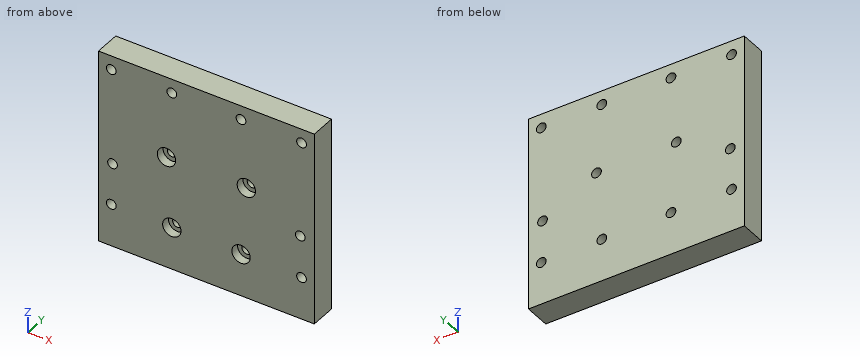
from build123d import *

# Parameters (mm, degrees)
SKETCH_W        = 100
SKETCH_H        = 90
PAD_DEPTH       = 12
SKETCH001_R     = 2.25
POCKET_DEPTH    = 12.001
SKETCH002_R     = 4.25
POCKET001_DEPTH = 4


with BuildPart() as part:
    # Sketch → Pad (new body)
    with BuildSketch(Plane.XZ):
        Rectangle(SKETCH_W, SKETCH_H)
    extrude(amount=PAD_DEPTH)

    # Sketch001 → Pocket (cut, through all)
    with BuildSketch(Plane.XZ.offset(12)):
        with Locations((-44.075, -25.33)):
            Circle(SKETCH001_R)
        with Locations((-43.5, -5.85)):
            Circle(SKETCH001_R)
        with Locations((-16.025, -25.33)):
            Circle(SKETCH001_R)
        with Locations((16.025, -25.33)):
            Circle(SKETCH001_R)
        with Locations((44.075, -25.33)):
            Circle(SKETCH001_R)
        with Locations((43.5, -5.85)):
            Circle(SKETCH001_R)
        with Locations((-44.075, 38.53)):
            Circle(SKETCH001_R)
        with Locations((-16.025, 38.53)):
            Circle(SKETCH001_R)
        with Locations((16.025, 38.53)):
            Circle(SKETCH001_R)
        with Locations((44.075, 38.53)):
            Circle(SKETCH001_R)
        with Locations((-18.5, 7.1)):
            Circle(SKETCH001_R)
        with Locations((18.5, 7.1)):
            Circle(SKETCH001_R)
    extrude(amount=-POCKET_DEPTH, mode=Mode.SUBTRACT)

    # Sketch002 → Pocket001 (cut)
    with BuildSketch(Plane.XZ.offset(12)):
        with Locations((-16.025, -25.33)):
            Circle(SKETCH002_R)
        with Locations((16.025, -25.33)):
            Circle(SKETCH002_R)
        with Locations((-18.5, 7.1)):
            Circle(SKETCH002_R)
        with Locations((18.5, 7.1)):
            Circle(SKETCH002_R)
    extrude(amount=-POCKET001_DEPTH, mode=Mode.SUBTRACT)


solid = part.part
For this review, take the finished solid that the model builds, in its own axes (mm). Round coordinates to 2 decimals unless told otherwise and drop trailing zeros. Loops run counter-clockwise (first coordinate to the right, second up) from the corner with the lowest first, then second, coordinate; pieces in that order, holes last. Notation, with made-up numbers: (50.25, 14) - (72.25, 14) arc R16 ccw to (72.25, 40) - close; hole circle Ø2 at (-15.5, -15.75). An arc over 180 degrees is marked (long way). Answer as CSV lines item,"result".
(1) Consider section B-B on y = -10.75. Give the number of separate pieces and of enclosed holes in the cut face, then the cut area to 3 significant figures.
Checked values:
separate pieces,"1"
enclosed holes,"12"
area,"8,650 mm2"
(2) Insertion check: P1, Ø3.5, axis at x = 44.075, z = 38.53, coming from the -Y side; P2, Ø2.5, axis at x = -20.5, z = 9, coming from the -Y side. Each pin has a flat end and moves straight along its axis. Give the tip position at first contact, or say it passes through.
Checked values:
P1,"passes through"
P2,"stops at y = -8"
(3) Wall thickness on line 1 (X direction, y = -9.25, z = -27); line 2 (Z direction, x = 18.5, y = -3.75); line 3 (Z direction, x = 18, y = -1.25): over which ranges is each line inside the solid? List them lowest first.
Checked values:
line 1,"x = -50 to -45.58, -42.57 to -19.93, -12.12 to 12.12, 19.93 to 42.57, 45.58 to 50"
line 2,"z = -45 to 4.85, 9.35 to 45"
line 3,"z = -45 to -26.41, -24.25 to 4.91, 9.29 to 37.45, 39.61 to 45"
(4) Consider section C-C on z = -5.85. Give the boundary of the cut face in (x, y).
Checked values:
outline,"(-50, -12) - (-45.75, -12) - (-45.75, 0) - (-50, 0) - close; (-41.25, -12) - (41.25, -12) - (41.25, 0) - (-41.25, 0) - close; (45.75, -12) - (50, -12) - (50, 0) - (45.75, 0) - close"
(5) Consider section A-A on z = -25.33. Give the boundary of the cut face in (x, y) (3 decimals).
Checked values:
outline,"(-50, -12) - (-46.325, -12) - (-46.325, 0) - (-50, 0) - close; (-41.825, -12) - (-20.275, -12) - (-20.275, -8) - (-18.275, -8) - (-18.275, 0) - (-41.825, 0) - close; (-13.775, -8) - (-11.775, -8) - (-11.775, -12) - (11.775, -12) - (11.775, -8) - (13.775, -8) - (13.775, 0) - (-13.775, 0) - close; (18.275, -8) - (20.275, -8) - (20.275, -12) - (41.825, -12) - (41.825, 0) - (18.275, 0) - close; (46.325, -12) - (50, -12) - (50, 0) - (46.325, 0) - close"
(6) Consider section D-D on x = 43.5. Give the boundary of the cut face in (y, z).
Checked values:
outline,"(-12, -45) - (0, -45) - (0, -27.51) - (-12, -27.51) - close; (-12, -23.15) - (0, -23.15) - (0, -8.1) - (-12, -8.1) - close; (-12, -3.6) - (0, -3.6) - (0, 36.35) - (-12, 36.35) - close; (-12, 40.71) - (0, 40.71) - (0, 45) - (-12, 45) - close"
